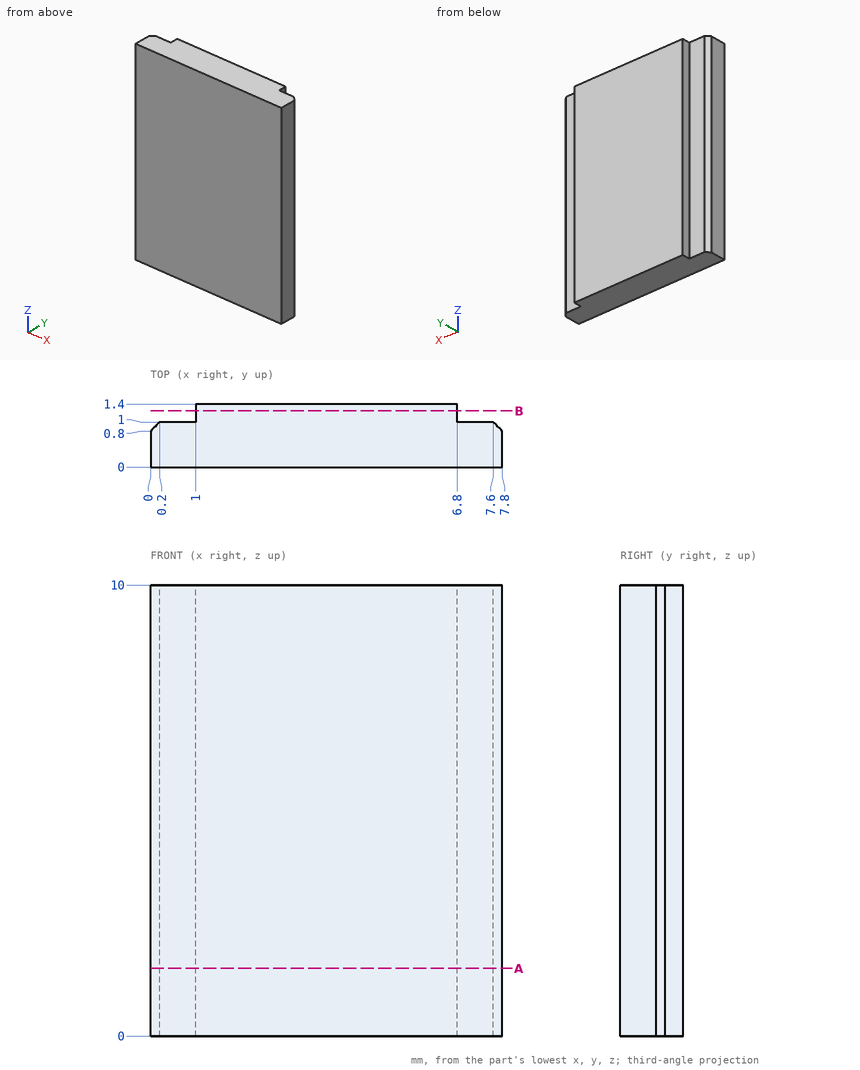
Here's the drawing with two shaded views (mm, measured from the low corner). I have some questions. Give positions to 0.01 mm unless a question says otherwise; leave off trailing zeros. Order: outer loops, then holes, each group sorted by start corner. A loop starts at its lowest first (then second) coordinate and runs counter-clockwise, first axis right, second up. Notation, with made-up numbers: (-34, -20) -> (-17, -20) arc R27 cw to (-17, -4) -> close; hole circle Ø9 at (38, -35.75). An arc over 180 degrees is marked (long way). Use a Markdown table: item, result. Add a question column.
Item 1: Imagine slicing it at A-A on z = 1.5. Please give me the cut outline in (x, y), plus the area to 3 significant figures.
Item 2: I need wall thicknesses on line 1 (Y direction, x = 0.5, z = 9.25); line 2 (X direction, y = 1.3, z = 1.25); line 3 (X direction, y = 0.95, z = 8.25). Which ranges of each line are inside material? Lowest first, please.
Item 3: Imagine slicing it at B-B on y = 1.25. Please give me the cut outline in (x, z), plus the area to 3 significant figures.
Data:
| question | item | result |
|---|---|---|
| 1 | outline | (0, 0) -> (7.8, 0) -> (7.8, 0.8) -> (7.6, 1) -> (6.8, 1) -> (6.8, 1.4) -> (1, 1.4) -> (1, 1) -> (0.2, 1) -> (0, 0.8) -> close |
| 1 | area | 10.1 mm² |
| 2 | line 1 | y = 0 to 1 |
| 2 | line 2 | x = 1 to 6.8 |
| 2 | line 3 | x = 0.15 to 7.65 |
| 3 | outline | (1, 0) -> (6.8, 0) -> (6.8, 10) -> (1, 10) -> close |
| 3 | area | 58.0 mm² |
